Design review of the part built by this model. Coordinates are the model's own, in mm. A direction names the side the tool comes from. Coordinates: 2 decimals unless noted, no trailing zeros. Loops run counter-clockwise (first coordinate to the right, second up) from the corner with the lowest first, then second, coordinate; pieces in that order, holes last. Notation, with made-up numbers: (-12.75, -27) - (8.25, -27) arc R25 ccw to (8.25, 7) - close; hole circle Ø6 at (5, 77). An arc over 180 degrees is marked (long way). Answer in a Markdown table with one row per item. Add a question column.
(1) Clearance check with flat-ended pins moving along their axes: pin 1 (4 mm diameter, centred on y = 84.5, z = -2.5, fed in from +X); pin 2 (6 mm diameter, centred on y = 86.5, z = -4, fed in from -X); pin 3 (5 mm diameter, centred on x = 5, y = 117.5, fed in from +Z). State where each tip first meets the part, or that it passes through.
(2) The part is to be moulded in two halves that separate along Z. For faces 1 (the face through (-3.955, 72.964, -5.158)), 2 (the face through (2, 148, 0)), 3 (the face through (0, 5, 0)), say which applies: released by +Z, released by -Z, zero draft, split by the parting line, or undercut.
(3) We need section B-B, the plane x = 0. Write out the cut boundary in (y, z).
(4) We need section C-C, the plane y = 89. Write out the cut boundary in (x, z), plus the area to 3 significant figures.
(5) For faces 4 (the face through (0, 143, 0)), 5 (the face through (2, 0, 0)), 6 (the face through (0.45, 2.53, 1.43)), list the 3-axis set-ups (+Z, -Z, +X, -X, +Y, -Y) from which the entire face can be reached by the end or side of a thin tool; tool diameter is ignored.
(6) To check wall thickness, follow L1, parallel to X at y = 144.45, z = 0; L2, parallel to Z at x = -0.5, y = 51; L3, parallel to X at y = 101, z = -0.25. State the ranges of each line that lie inside material, in increasing order. Write a range as [from, to].
(7) We need section A-A, the plane z = 0. Write out the cut boundary in (x, y), plus the area to 3 significant figures.
from build123d import *

# Parameters (mm, degrees)
SKETCH1_R           = 6.5
BOSS_EXTRUDE1_DEPTH = 148
SKETCH2_R           = 1.5
CUT_EXTRUDE1_DEPTH  = 5
LPATTERN1_COUNT     = 2
LPATTERN1_PITCH     = 143


with BuildPart() as part:
    # Sketch1 → Boss-Extrude1 (new body)
    with BuildSketch(Plane(origin=(0, 0, 0), x_dir=(1, 0, 0), z_dir=(0, 1, 0))):
        with Locations(Location((0, 0, 0), (0, 0, 270))):
            Circle(SKETCH1_R)
    extrude(amount=BOSS_EXTRUDE1_DEPTH)

    # Sketch2 → Cut-Extrude1 (cut)
    with BuildSketch(Plane(origin=(0, 148, 0), x_dir=(1, 0, 0), z_dir=(0, 1, 0))):
        with Locations(Location((0, 0, 0), (0, 0, 270))):
            Circle(SKETCH2_R)
    cut_extrude1 = extrude(amount=-CUT_EXTRUDE1_DEPTH, mode=Mode.SUBTRACT)

    # LPattern1: Cut-Extrude1 ×2
    with Locations(*[(0, -i * LPATTERN1_PITCH, 0) for i in range(1, LPATTERN1_COUNT)]):
        add(cut_extrude1, mode=Mode.SUBTRACT)


solid = part.part
Responses:
| question | item | result |
|---|---|---|
| 1 | pin 1 | stops at x = 6.48 |
| 1 | pin 2 | stops at x = -6.42 |
| 1 | pin 3 | stops at z = 6 |
| 2 | face 1 | split by the parting line |
| 2 | face 2 | zero draft |
| 2 | face 3 | undercut |
| 3 | outline | (0, -6.5) - (148, -6.5) - (148, -1.5) - (143, -1.5) - (143, 1.5) - (148, 1.5) - (148, 6.5) - (0, 6.5) - (0, 1.5) - (5, 1.5) - (5, -1.5) - (0, -1.5) - close |
| 4 | outline | circle Ø13 at (0, 0) |
| 4 | area | 133 mm2 |
| 5 | face 4 | +Y |
| 5 | face 5 | +Z, -Z, +X, -X, -Y |
| 5 | face 6 | -Y |
| 6 | L1 | x = [-6.5, -1.5], [1.5, 6.5] |
| 6 | L2 | z = [-6.48, 6.48] |
| 6 | L3 | x = [-6.5, 6.5] |
| 7 | outline | (-6.5, 0) - (-1.5, 0) - (-1.5, 5) - (1.5, 5) - (1.5, 0) - (6.5, 0) - (6.5, 148) - (1.5, 148) - (1.5, 143) - (-1.5, 143) - (-1.5, 148) - (-6.5, 148) - close |
| 7 | area | 1,890 mm2 |
